from build123d import *

# Parameters (mm, degrees)
SKETCH1_R               = 4.064
BOSS_EXTRUDE1_DEPTH     = 32.512
SKETCH2_W               = 26.416
SKETCH2_H               = 40.132
CUT_EXTRUDE1_DEPTH      = 59.42
SKETCH3_R               = 4.125
CUT_EXTRUDE3_DEPTH      = 44.18
CUT_EXTRUDE3_DEPTH_BACK = 35.052


with BuildPart() as part:
    # Sketch1 → Boss-Extrude1 (new body)
    with BuildSketch(Plane(origin=(0, 0, 0), x_dir=(0, 0, -1), z_dir=(1, 0, 0))):
        with BuildLine():
            Line((0, 16.002), (45.896514256, 42.085387724))
            ThreePointArc((45.896514256, 42.085387724), (54.253684434, 42.0427173), (58.42, 34.798))
            Line((58.42, 34.798), (58.42, 0))
            Line((58.42, 0), (0, 0))
            Line((0, 0), (0, 16.002))
        make_face()
        with Locations((50.038, 34.798)):
            Circle(SKETCH1_R, mode=Mode.SUBTRACT)
    extrude(amount=-BOSS_EXTRUDE1_DEPTH)

    # Sketch2 → Cut-Extrude1 (cut, through all)
    with BuildSketch(Plane.XY):
        with Locations((-16.256, 23.114)):
            Rectangle(SKETCH2_W, SKETCH2_H)
    extrude(amount=-CUT_EXTRUDE1_DEPTH, mode=Mode.SUBTRACT)

    # Sketch3 → Cut-Extrude3 (cut, two sides)
    with BuildSketch(Plane(origin=(0, 0, 0), x_dir=(1, 0, 0), z_dir=(0, 1, 0))) as cut_extrude3_sk:
        with Locations(Location((-16.256, 12, 0), (0, 0, 90))):  # turned: the seam where the file's is
            Circle(SKETCH3_R)
        with BuildLine():
            Line((-20.574, 48.42), (-20.574, 58.42))
            Line((-20.574, 58.42), (-11.938, 58.42))
            Line((-11.938, 58.42), (-11.938, 48.42))
            ThreePointArc((-11.938, 48.42), (-16.256, 44.102), (-20.574, 48.42))
        make_face()
    extrude(amount=CUT_EXTRUDE3_DEPTH, mode=Mode.SUBTRACT)
    extrude(cut_extrude3_sk.sketch, amount=-CUT_EXTRUDE3_DEPTH_BACK, mode=Mode.SUBTRACT)


solid = part.part
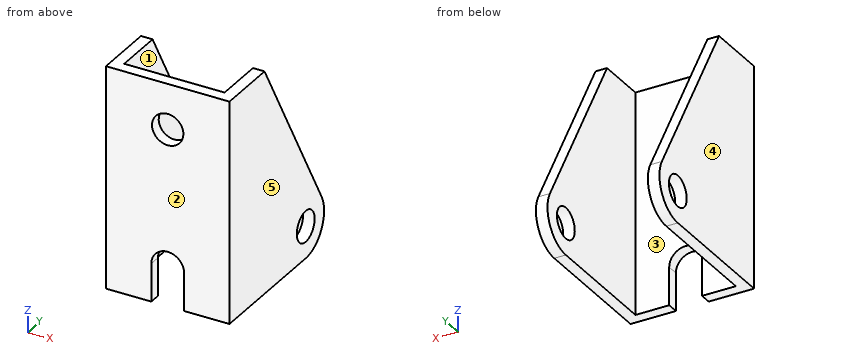
Geometry: final body of the model. Coordinates: model frame, mm. Face numbers are marked on the shaded views. A direction names the side the tool comes from. Coordinates: 2 decimals unless noted, no trailing zeros. Loops run counter-clockwise (first coordinate to the right, second up) from the corner with the lowest first, then second, coordinate; pieces in that order, holes last. Notation, with made-up numbers: M 34.5,58 L 64.5,58 A20 cw 64.5,88 Z; hole C 34.5,17.5 d4. An arc over 180 degrees is marked long. One line per item, written item: value. Start each with the question number.
1) Pin query (flat end, axial travel): P1, Ø10.5, axis at x = -16.256, z = -12, coming from the +Y side; P2, Ø5, axis at y = 34.798, z = -50.038, coming from the -X side; P3, Ø5, axis at x = -29, y = 27.5, coming from the +Z side; P4, Ø12, axis at x = -18.5, z = -48.5, coming from the -Y side. Return the tip coordinate at first contact, or that it passes through.
2) Material intervals for L1, parallel to X at y = 20.5, z = -12.5; L2, parallel to Y at x = -15, z = -33; L3, parallel to Y at x = -30, z = -34, sorted ascending. Write a range as from..to.
3) Cut plane A-A (y = 24). Return loops of the section in (x, z).
4) Cut plane B-B (z = -12). Return loops of the section in (x, y).
5) Draft query along X for the marked faces 3, 4 and 5. Return one class per face: released by +X, released by -X, zero draft, split by the parting line, or undercut.
6) Cut plane D-D (z = -50). Return loops of the section in (x, y), then the cut area to 3 significant figures.
7) Reachability of the marked faces 1 and 2 from +Z, -Z, +X, -X, +Y, -Y: full face, straight path, thin tool, end or side. Return the list, or none.
8) Cut plane C-C (x = -19). Return loops of the section in (y, z), then the cut area to 3 significant figures.
Evaluation:
1. P1: y = 3.05
1. P2: through
1. P3: z = -15.91
1. P4: y = 0
2. L1: -32.51..-29.46, -3.05..0
2. L2: 0..3.05
2. L3: 0..35.32
3. outline: M -32.51,-58.42 L -29.46,-58.42 L -29.46,-14.07 L -32.51,-14.07 Z; M -3.05,-58.42 L 0,-58.42 L 0,-14.07 L -3.05,-14.07 Z
4. outline: M -32.51,0 L -20.38,0 L -20.38,3.05 L -29.46,3.05 L -29.46,22.82 L -32.51,22.82 Z; M -12.13,0 L 0,0 L 0,22.82 L -3.05,22.82 L -3.05,3.05 L -12.13,3.05 Z
5. face 3: undercut
5. face 4: released by -X
5. face 5: released by +X
6. outline: M -32.51,0 L -20.57,0 L -20.57,3.05 L -29.46,3.05 L -29.46,30.73 L -32.51,30.73 Z; M -32.51,38.86 L -29.46,38.86 L -29.46,43.18 L -32.51,43.18 Z; M -11.94,0 L 0,0 L 0,30.73 L -3.05,30.73 L -3.05,3.05 L -11.94,3.05 Z; M -3.05,38.86 L 0,38.86 L 0,43.18 L -3.05,43.18 Z
6. area: 268 mm^2
7. face 1: +Z, -Z, +Y
7. face 2: +Z, -Z, +X, -X, -Y
8. outline: M 0,-45.09 L 3.05,-45.09 L 3.05,-15.08 L 0,-15.08 Z; M 0,-8.92 L 3.05,-8.92 L 3.05,0 L 0,0 Z
8. area: 119 mm^2
